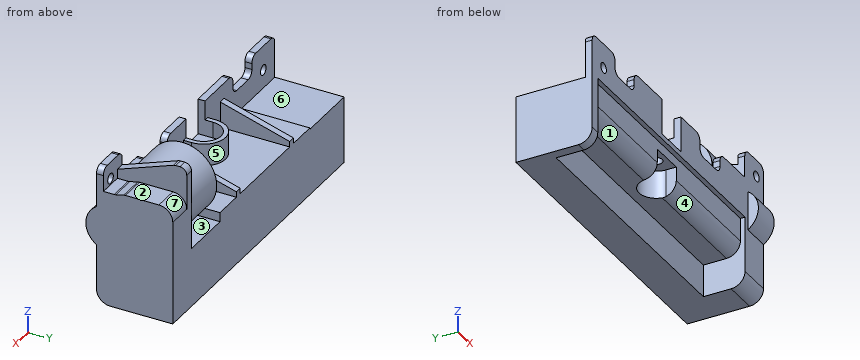
from build123d import *

# Parameters (mm, degrees)
EXTRUDE_1_DEPTH          = 1.5
EXTRUDE_2_DEPTH          = 16.5
EXTRUDE_START            = 36.3
EXTRUDE_3_DEPTH          = 6.2
EXTRUDE_START_2          = 28.9
EXTRUDE_4_DEPTH          = 1.9
CUT_EXTRUDE_START        = 36.3
CUT_EXTRUDE_1_DEPTH      = 5.5
SKETCH_3_6_R             = 7.45
EXTRUDE_7_DEPTH          = 10
FILLET_1_R               = 1.5
FILLET_2_R               = 1.5
FILLET_3_R               = 1.5
FILLET_4_R               = 3
EXTRUDE_START_3          = -4.7
EXTRUDE_5_DEPTH          = 4.8
CUT_EXTRUDE_START_2      = -3.4
CUT_EXTRUDE_2_OUTLINE_W  = 7.5
CUT_EXTRUDE_2_OUTLINE_H  = 1.5
CUT_EXTRUDE_2_DEPTH      = 0.5
EXTRUDE_6_DEPTH          = 1.3
CUT_EXTRUDE_START_3      = -19.5
CUT_EXTRUDE_3_DEPTH      = 13
CUT_EXTRUDE_4_DEPTH      = 44.001744151
CUT_EXTRUDE_4_DEPTH_BACK = 44.001744151
SKETCH_5_R               = 1.25
EXTRUDE_START_4          = 9.75
EXTRUDE_8_DEPTH          = 1.5
EXTRUDE_START_5          = -9.75
EXTRUDE_9_DEPTH          = 1.5
SKETCH_7_W               = 29
SKETCH_7_H               = 7
CUT_EXTRUDE_5_DEPTH      = 9
SKETCH_7_3_W             = 29
SKETCH_7_3_H             = 8
CUT_EXTRUDE_6_DEPTH      = 1
FILLET_5_R               = 3
FILLET_6_R               = 3
SKETCH_1_4_R             = 1.1
CUT_EXTRUDE_7_DEPTH      = 2


# Read off the part's stored shape, not the designer's step: Бобышка-Вытянуть5, Вырез-Вытянуть2, Бобышка-Вытянуть6, Вырез-Вытянуть3
with BuildPart() as part:
    # Эскиз1 → Бобышка-Вытянуть1 (new body)
    with BuildSketch(Plane(origin=(0, 0, 0), x_dir=(1, 0, 0), z_dir=(0, 1, 0))):
        Polygon((36.3, 19.5), (-31.2, 19.5), (-31.2, -4.3), (-22.2, -4.3), (-22.2, 0), (-14.7, 0), (-14.7, -4.3), (-3.75, -4.3), (-3.75, 2.9), (3.75, 2.9), (3.75, -4.3), (11.25, -4.3), (11.25, 0), (19.15, 0), (19.15, -4.3), (28.9, -4.3), (28.9, -10.5), (36.3, -10.5), align=None)
    extrude(amount=EXTRUDE_1_DEPTH)

    # Эскиз1<3> → Бобышка-Вытянуть2 (add)
    with BuildSketch(Plane(origin=(0, 0, 0), x_dir=(1, 0, 0), z_dir=(0, 1, 0))):
        Polygon((36.3, 19.5), (-31.2, 19.5), (-31.2, 5), (-17.7, 5), (-17.7, 4.7), (17.7, 4.7), (17.7, 6.7), (28.9, 6.7), (28.9, -6), (36.3, -6), align=None)
    extrude(amount=EXTRUDE_2_DEPTH)

    # Эскиз3 → Бобышка-Вытянуть3 (add)
    with BuildSketch(Plane(origin=(0, 0, 0), x_dir=(0, 0, -1), z_dir=(1, 0, 0)).offset(EXTRUDE_START)):
        with BuildLine():
            Line((0, 1.5), (0, 0))
            Line((0, 0), (6.708325083, 0))
            ThreePointArc((6.708325083, 0), (7.092746426, 0.723467616), (7.35386444, 1.5))
            Line((7.35386444, 1.5), (0, 1.5))
        make_face()
        with BuildLine():
            Line((6.708325083, 0), (0, 0))
            Line((0, 0), (0, 1.5))
            Line((0, 1.5), (-2.35386444, 1.5))
            ThreePointArc((-2.35386444, 1.5), (1.683495092, -2.232881484), (6.708325083, 0))
        make_face()
    extrude(amount=-EXTRUDE_3_DEPTH)

    # Эскиз3<4> → Бобышка-Вытянуть4 (add)
    with BuildSketch(Plane(origin=(0, 0, 0), x_dir=(0, 0, -1), z_dir=(1, 0, 0)).offset(EXTRUDE_START_2)):
        Polygon((-7.5, 1.5), (-6, 1.5), (-6, 16.5), (-12, 16.5), (-12, 13.863648388), align=None)
    extrude(amount=EXTRUDE_4_DEPTH)

    # Эскиз3<5> → Вырез-Вытянуть1 (cut)
    with BuildSketch(Plane(origin=(0, 0, 0), x_dir=(0, 0, -1), z_dir=(1, 0, 0)).offset(CUT_EXTRUDE_START)):
        Polygon((-6, 1.5), (-5.5, 1.5), (-5.5, 4), (-6, 6.078204319), align=None)
    extrude(amount=-CUT_EXTRUDE_1_DEPTH, mode=Mode.SUBTRACT)

    # Эскиз3<6> → Бобышка-Вытянуть7 (add)
    with BuildSketch(Plane(origin=(0, 0, 0), x_dir=(0, 0, -1), z_dir=(1, 0, 0)).offset(EXTRUDE_START_2)):
        with Locations((-1.9, 9)):
            Circle(SKETCH_3_6_R)
    extrude(amount=-EXTRUDE_7_DEPTH)

    # Скругление1
    fillet_1_edges = [part.edges().sort_by_distance(p)[0] for p in [
        (36.3, 0.75, 10.5),
        (28.9, 0.75, 10.5),
        (19.15, 0.75, 4.3),
        (19.15, 0.75, 0),
        (11.25, 0.75, 0),
        (11.25, 0.75, 4.3),
        (-14.7, 0.75, 4.3),
        (-14.7, 0.75, 0),
        (-22.2, 0.75, 0),
        (-22.2, 0.75, 4.3),
        (-31.2, 0.75, 4.3),
    ]]
    fillet(fillet_1_edges, radius=FILLET_1_R)

    # Скругление2
    fillet_2_edges = [part.edges().sort_by_distance(p)[0] for p in [
        (29.85, 16.5, 12),
        (29.85, 13.863648388, 12),
    ]]
    fillet(fillet_2_edges, radius=FILLET_2_R)

    # Скругление3
    fillet_3_edges = [part.edges().sort_by_distance(p)[0] for p in [
        (33.55, 6.078204319, 6),
        (33.55, 4, 5.5),
    ]]
    fillet(fillet_3_edges, radius=FILLET_3_R)

    # Скругление4
    fillet_4_edges = [part.edges().sort_by_distance(p)[0] for p in [
        (33.55, 16.5, 6),
    ]]
    fillet(fillet_4_edges, radius=FILLET_4_R)

    # Бобышка-Вытянуть5 outline → Бобышка-Вытянуть5 (add)
    with BuildSketch(Plane.XY.offset(EXTRUDE_START_3)):
        with BuildLine():
            Line((-3.75, 1.5), (-3.75, 3.25))
            ThreePointArc((-3.75, 3.25), (0, 7), (3.75, 3.25))
            Line((3.75, 3.25), (3.75, 1.5))
            Line((3.75, 1.5), (4.75, 1.5))
            Line((4.75, 1.5), (4.75, 3.25))
            ThreePointArc((4.75, 3.25), (0, 8), (-4.75, 3.25))
            Line((-4.75, 3.25), (-4.75, 1.5))
            Line((-4.75, 1.5), (-3.75, 1.5))
        make_face()
    extrude(amount=EXTRUDE_5_DEPTH)

    # Вырез-Вытянуть2 outline → Вырез-Вытянуть2 (cut)
    with BuildSketch(Plane.XY.offset(CUT_EXTRUDE_START_2)):
        with Locations((0, 0.75)):
            Rectangle(CUT_EXTRUDE_2_OUTLINE_W, CUT_EXTRUDE_2_OUTLINE_H)
    extrude(amount=CUT_EXTRUDE_2_DEPTH, mode=Mode.SUBTRACT)

    # Бобышка-Вытянуть6 outline → Бобышка-Вытянуть6 (add)
    with BuildSketch(Plane.XY.offset(EXTRUDE_START_3)):
        with BuildLine():
            Line((-3.75, 1.5), (3.75, 1.5))
            Line((3.75, 1.5), (3.75, 3.25))
            ThreePointArc((3.75, 3.25), (0, 7), (-3.75, 3.25))
            Line((-3.75, 3.25), (-3.75, 1.5))
        make_face()
    extrude(amount=EXTRUDE_6_DEPTH)

    # Вырез-Вытянуть3 outline → Вырез-Вытянуть3 (cut)
    with BuildSketch(Plane.XY.offset(CUT_EXTRUDE_START_3)):
        with BuildLine():
            Line((-3.75, 3.25), (-3.75, 0))
            Line((-3.75, 0), (3.75, 0))
            Line((3.75, 0), (3.75, 3.25))
            ThreePointArc((3.75, 3.25), (0, 7), (-3.75, 3.25))
        make_face()
    extrude(amount=CUT_EXTRUDE_3_DEPTH, mode=Mode.SUBTRACT)

    # Эскиз5 → Вырез-Вытянуть4 (cut, two sides: drawn at the far end of the back side and taken through both)
    with BuildSketch(Plane.XY.offset(-3.4).offset(-CUT_EXTRUDE_4_DEPTH_BACK)):
        with Locations((0, 3.25)):
            Circle(SKETCH_5_R)
    extrude(amount=CUT_EXTRUDE_4_DEPTH + CUT_EXTRUDE_4_DEPTH_BACK, mode=Mode.SUBTRACT)

    # Эскиз6 → Бобышка-Вытянуть8 (add)
    with BuildSketch(Plane(origin=(0, 0, 0), x_dir=(0, 0, -1), z_dir=(1, 0, 0)).offset(EXTRUDE_START_4)):
        Polygon((4.7, 1.5), (4.7, 16.5), (3.5, 16.5), (-0.9, 1.5), align=None)
    extrude(amount=EXTRUDE_8_DEPTH)

    # Эскиз6<4> → Бобышка-Вытянуть9 (add)
    with BuildSketch(Plane(origin=(0, 0, 0), x_dir=(0, 0, -1), z_dir=(1, 0, 0)).offset(EXTRUDE_START_5)):
        Polygon((4.7, 1.5), (4.7, 16.5), (3.5, 16.5), (-0.9, 1.5), align=None)
    extrude(amount=-EXTRUDE_9_DEPTH)

    # Эскиз7 → Вырез-Вытянуть5 (cut)
    with BuildSketch(Plane(origin=(0, 0, 0), x_dir=(1, 0, 0), z_dir=(0, 1, 0))):
        with Locations((14.5, 16)):
            Rectangle(SKETCH_7_W, SKETCH_7_H)
        with Locations((-14.5, 16)):
            Rectangle(SKETCH_7_W, SKETCH_7_H)
    extrude(amount=CUT_EXTRUDE_5_DEPTH, mode=Mode.SUBTRACT)

    # Эскиз7<3> → Вырез-Вытянуть6 (cut)
    with BuildSketch(Plane(origin=(0, 0, 0), x_dir=(1, 0, 0), z_dir=(0, 1, 0))):
        with Locations((14.5, 8.5)):
            Rectangle(SKETCH_7_3_W, SKETCH_7_3_H)
        with Locations((-14.5, 8.5)):
            Rectangle(SKETCH_7_3_W, SKETCH_7_3_H)
    extrude(amount=CUT_EXTRUDE_6_DEPTH, mode=Mode.SUBTRACT)

    # Скругление5
    fillet_5_edges = [part.edges().sort_by_distance(p)[0] for p in [
        (-16.375, 1, -12.5),
        (16.375, 1, -12.5),
    ]]
    fillet(fillet_5_edges, radius=FILLET_5_R)

    # Скругление6
    fillet_6_edges = [part.edges().sort_by_distance(p)[0] for p in [
        (-30.1, 0, -19.5),
        (32.65, 0, -19.5),
    ]]
    fillet(fillet_6_edges, radius=FILLET_6_R)

    # Эскиз1<4> → Вырез-Вытянуть7 (cut)
    with BuildSketch(Plane(origin=(0, 0, 0), x_dir=(1, 0, 0), z_dir=(0, 1, 0))):
        with Locations(Location((-26.7, 1, 0), (0, 0, 270))):
            Circle(SKETCH_1_4_R)
        with Locations(Location((33.5, -6.9, 0), (0, 0, 270))):
            Circle(SKETCH_1_4_R)
    extrude(amount=CUT_EXTRUDE_7_DEPTH, mode=Mode.SUBTRACT)


solid = part.part
Input: part model. Units: mm. Frame: model coordinates. Face numbers are marked on the shaded views. A direction names the side the tool comes from. Give positions to 0.01 mm unless a question says otherwise; leave off trailing zeros. Order: outer loops, then holes, each group sorted by start corner. A loop starts at its lowest first (then second) coordinate and runs counter-clockwise, first axis right, second up.
Q1. Draft query along X for the marked faces 1 and 2. Return one class per face: +X half, -X half, draft (parallel to the pull), parting line (faces both ways), or undercut.
Checked values:
face 1: undercut
face 2: draft
Q2. Section A-A on x = 33.5. Output: boundary loops of the cut face in (y, z).
Checked values:
outline: (0, -16.5) arc R3 ccw to (3, -19.5) - (16.5, -19.5) - (16.5, 3) arc R3 ccw to (13.5, 6) - (6.26, 6) arc R1.5 ccw to (5.91, 5.96) - (4.17, 5.54) arc R1.5 cw to (3.82, 5.5) - (1.5, 5.5) - (1.5, 5.8) - (0, 5.8) - (0, 1.71) arc R5 ccw to (0, -6.71) - close; (0, 8) - (1.5, 8) - (1.5, 10.5) - (0, 10.5) - close
Q3. Set-up query: the marked faces 3, 4, 5, 6 and 7. Return all of +Z, -Z, +X, -X, +Y, -Y with unobstructed straight access to the full face (end or side cutting, diameter ignored); none if empty.
Checked values:
face 3: +Y
face 4: -Z, -Y
face 5: +Z, +Y
face 6: +Z, -X, +Y
face 7: +Z, +X, +Y
Q4. Section C-C on x = 0. Output: boundary loops of the cut face in (y, z).
Checked values:
outline: (0, -4.5) - (1, -4.5) - (1, -6.5) - (2, -6.5) - (2, -3.4) - (0, -3.4) - close; (4.5, -6.5) - (7, -6.5) - (7, -12.5) - (9, -12.5) - (9, -19.5) - (16.5, -19.5) - (16.5, -4.7) - (8, -4.7) - (8, 0.1) - (7, 0.1) - (7, -3.4) - (4.5, -3.4) - close
Q5. Contact query for flat-ended pins moving along their axis: pin 1 Ø0.8 at (x, y) = (-9.5, 0.5) entering from +Z; pin 2 Ø0.8 at (x, y) = (16, 0.5) entering from +Z; pin 3 Ø1.5 at (x, z) = (-24, -13.5) entering from -Y. Output: stop coordinate, or through.
Checked values:
pin 1: stops at z = 4.3
pin 2: stops at z = 0
pin 3: stops at y = 9
Q6. Section D-D on y = 10.75. Output: boundary loops of the cut face in (x, z), and give its area (3 significant figures).
Checked values:
outline: (-31.2, -19.5) - (36.3, -19.5) - (36.3, 6) - (30.8, 6) - (30.8, 10.87) - (28.9, 10.87) - (28.9, 9.14) - (18.9, 9.14) - (18.9, -5.34) - (28.9, -5.34) - (28.9, -6.7) - (17.7, -6.7) - (17.7, -4.7) - (11.25, -4.7) - (11.25, -1.81) - (9.75, -1.81) - (9.75, -4.7) - (-9.75, -4.7) - (-9.75, -1.81) - (-11.25, -1.81) - (-11.25, -4.7) - (-17.7, -4.7) - (-17.7, -5) - (-31.2, -5) - close
area: 1,210 mm2
Q7. Ray query, probe 1 along X at (y, z) = (3.25, -4.5); probe 2 along Y at (x, z) = (0, -4); probe 3 along Z at (x, y) = (-26.7, 0.6). Return the intervals inside material, ascending.
Checked values:
probe 1: x = -11.25 to -9.75, -4.75 to -1.25, 1.25 to 4.75, 9.75 to 11.25, 28.9 to 36.3
probe 2: y = 0 to 2, 4.5 to 8
probe 3: z = -4.5 to -2.1, 0.1 to 4.3
